Source: CAD feature listing. Evaluate the final solid. Frame: model axes, mm. A direction names the side the tool comes from. Give positions to 0.01 mm unless a question says otherwise; leave off trailing zeros. Put each result on its own line as item: value.
```python
from build123d import *


with BuildPart() as part:
    # Schizzo1 → Rivoluzione1 (revolve)
    with BuildSketch(Plane(origin=(0, 0, 0), x_dir=(0, 0, -1), z_dir=(1, 0, 0)), mode=Mode.PRIVATE) as rivoluzione1_sk:
        with BuildLine():
            Line((-13.75, -3.75297619), (-11.815, -1.28797619))
            Line((-11.815, -1.28797619), (-9.495, -1.28797619))
            Line((-9.495, -1.28797619), (-9.495, 1.38202381))
            Line((-9.495, 1.38202381), (-4.645, 1.38202381))
            Line((-4.645, 1.38202381), (-4.645, -1.61797619))
            Line((-4.645, -1.61797619), (-10.241809827, -2.522914521))
            Line((-10.241809827, -2.522914521), (-11.525724899, -4.158496253))
            ThreePointArc((-11.525724899, -4.158496253), (-7.042068941, -10.027197542), (0, -12.25297619))
            ThreePointArc((0, -12.25297619), (7.042068941, -10.027197542), (11.525724899, -4.158496253))
            Line((11.525724899, -4.158496253), (10.241809827, -2.522914521))
            Line((10.241809827, -2.522914521), (4.645, -1.61797619))
            Line((4.645, -1.61797619), (4.645, 1.38202381))
            Line((4.645, 1.38202381), (9.495, 1.38202381))
            Line((9.495, 1.38202381), (9.495, -1.28797619))
            Line((9.495, -1.28797619), (11.815, -1.28797619))
            Line((11.815, -1.28797619), (13.75, -3.75297619))
            ThreePointArc((13.75, -3.75297619), (8.650325138, -11.327806729), (0, -14.25297619))
            ThreePointArc((0, -14.25297619), (-8.650325138, -11.327806729), (-13.75, -3.75297619))
        make_face()
    revolve(rivoluzione1_sk.sketch.rotate(Axis((0, 40.99702381, 83.136994768), (0, 0, -1)), 270), axis=Axis((0, 40.99702381, 83.136994768), (0, 0, -1)))


solid = part.part
```
(1) Line query: probe 1 along Y at (x, z) = (0, 5.9); probe 2 along X at (y, z) = (4.5, 6.5); probe 3 along Y at (x, z) = (0, 6.2). Output: solid intervals per line, ascending. Write a range as from..to.
Calculated:
probe 1: y = -12.97..-10.74, -1.82..1.38, 80.61..83.81, 92.73..94.97
probe 2: x = -39.37..-36.17, -22.58..-15.41, 15.41..22.58, 36.17..39.37
probe 3: y = -12.83..-10.57, -1.87..1.38, 80.61..83.86, 92.56..94.83
(2) Reachability of faces 1 (the cylindrical face through (19.51, 78.51, -10.67)), 2 (the cylindrical face through (19.51, 78.51, 10.64)), 3 (the cylindrical face through (21.297, 7.594, -7.104)), 4 (the flat face through (12, 79, -4.645)) from +Z, -Z, +X, -X, +Y, -Y: full face, straight path, thin tool, end or side. Return the list, or none.
Calculated:
face 1: -Z
face 2: +Z
face 3: +Z, -Z
face 4: none
(3) First-contact query: P1, Ø5, axis at x = 20, z = -1.5, coming from the +Y side; P2, Ø6, axis at y = 62.5, z = 4, coming from the -X side; P3, Ø12, axis at y = 2, z = 6.5, coming from the +X side. Flat tips, straight axial feed; report the tip coordinate or a pass-through.
Calculated:
P1: stops at y = 93.35
P2: stops at x = -51.68
P3: stops at x = 43.18
